Part print with two shaded views. Sizes in mm from the minimum x, y, z corner. A direction names the side the tool comes from. Round coordinates to 2 decimals unless told otherwise and drop trailing zeros. Loops run counter-clockwise (first coordinate to the right, second up) from the corner with the lowest first, then second, coordinate; pieces in that order, holes last.
(1) Cut at D-D on y = 34. List the corners of the cut face in (x, z).
(2) Tool access for the marked faces 1, 2, 3 and 4: list every direction of +Z, -Z, +X, -X, +Y, -Y with a clear straight run to the whole face (end or side of a thin tool).
(3) Cut at C-C on z = 15.75. List the corners of the cut face in (x, y).
(4) Flat gauge pins, fed straight in: pin 1 (4.5 mm diameter, centred on x = 43.5, z = 13.5, fed in from +Y); pin 2 (4 mm diameter, centred on x = 3, y = 3.25, fed in from -Z); pin 3 (10 mm diameter, centred on x = 15, y = 37.5, fed in from +Z); pin 4 (6 mm diameter, centred on x = 39.5, y = 11.5, fed in from +Z). Where does each tip first touch, or does it go through?
(5) Probe probe 1 along Y at (x, z) = (3, 1.1); probe 2 along Z at (x, y) = (21.5, 21.5); probe 3 along X at (y, z) = (23.5, 6). List the from-to ranges inside material, lowest first.
(6) Cut at A-A on x = 67. List the corners of the cut face in (y, z), then the cut area to 3 significant figures.
(7) Cut at B-B on y = 3.25. List the corners of the cut face in (x, z), then the cut area to 3 significant figures.
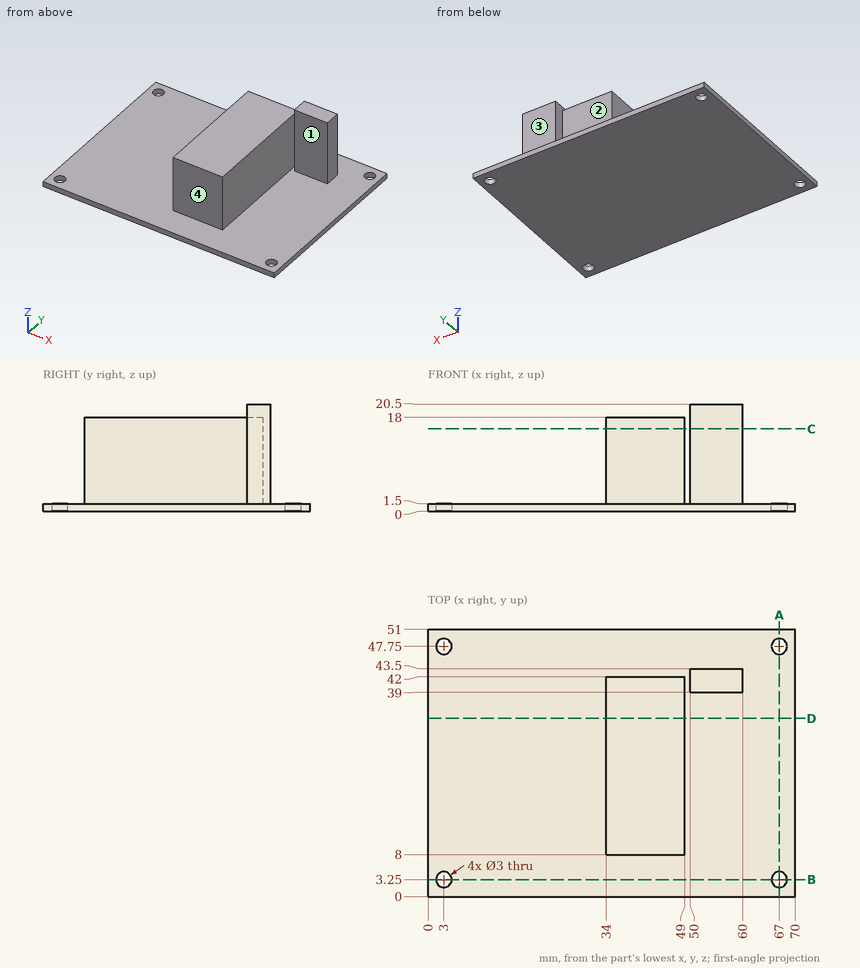
Final values:
1. outline: (0, 0) - (70, 0) - (70, 1.5) - (49, 1.5) - (49, 18) - (34, 18) - (34, 1.5) - (0, 1.5) - close
2. face 1: +Z, +X, -Y
2. face 2: +Z, -X, +Y
2. face 3: +Z, +X, -X, +Y
2. face 4: +Z, +X, -X, -Y
3. outline: (34, 8) - (49, 8) - (49, 42) - (34, 42) - close; (50, 39) - (60, 39) - (60, 43.5) - (50, 43.5) - close
4. pin 1: stops at y = 42
4. pin 2: stops at z = 0
4. pin 3: stops at z = 1.5
4. pin 4: stops at z = 18
5. probe 1: y = 0 to 1.75, 4.75 to 46.25, 49.25 to 51
5. probe 2: z = 0 to 1.5
5. probe 3: x = 34 to 49
6. outline: (0, 0) - (1.75, 0) - (1.75, 1.5) - (0, 1.5) - close; (4.75, 0) - (46.25, 0) - (46.25, 1.5) - (4.75, 1.5) - close; (49.25, 0) - (51, 0) - (51, 1.5) - (49.25, 1.5) - close
6. area: 67.5 mm2
7. outline: (0, 0) - (1.5, 0) - (1.5, 1.5) - (0, 1.5) - close; (4.5, 0) - (65.5, 0) - (65.5, 1.5) - (4.5, 1.5) - close; (68.5, 0) - (70, 0) - (70, 1.5) - (68.5, 1.5) - close
7. area: 96.0 mm2
